```python
from build123d import *

# Parameters (mm, degrees)
F0_W        = 600
F0_H        = 700
F1_DEPTH    = 800
F2_W        = 700
F2_H        = 80
F3_DEPTH    = 25
F5_DEPTH    = 50
F6_T1_DEPTH = 120
F6_T4_ANGLE = 180
F6_T6_ANGLE = 180
F7_W        = 40
F7_H        = 110
F8_DEPTH    = 25
F9_R        = 4.99999
F10_W       = 630
F10_H       = 700
F11_DEPTH   = 25


# Not quite as in the source:
# - a fillet or chamfer that OpenCascade refuses, or shapes differently, is made with other operations: its cross-section is extruded or revolved along the edge and cut away or added
# - a fillet or chamfer is up to 0.001 mm smaller than in the source, because OpenCascade refuses the exact size


with BuildPart() as f1:
    # F0 (on Top) → F1 (new body)
    with BuildSketch(Plane.XY):
        Rectangle(F0_W, F0_H)
    extrude(amount=F1_DEPTH)

    # F2 (on face) → F3 (cut)
    with BuildSketch(Plane.YZ.offset(300)):
        with Locations((0, 40)):
            Rectangle(F2_W, F2_H)
    extrude(amount=-F3_DEPTH, mode=Mode.SUBTRACT)

    # F4 (on face) → F5 (join)
    with BuildSketch(Plane.YZ.offset(300)):
        with BuildLine():
            ThreePointArc((-320, 750), (-323.5355339059, 748.5355339059), (-325, 745))
            Line((-325, 745), (-325, 625))
            ThreePointArc((-325, 625), (-323.5355339059, 621.4644660941), (-320, 620))
            ThreePointArc((-320, 620), (-316.4644660941, 621.4644660941), (-315, 625))
            Line((-315, 625), (-315, 745))
            ThreePointArc((-315, 745), (-316.4644660941, 748.5355339059), (-320, 750))
        make_face()
    extrude(amount=F5_DEPTH)

    # F6: fillet of radius 5 on 4 edges, made by hand

    # F6_s2 → F6_t1 (cut)
    with BuildSketch(Plane.XY.offset(625)):
        with BuildLine():
            ThreePointArc((345, -325), (348.5355339059, -323.5355339059), (350, -320))
            Line((350, -320), (350, -325))
            Line((350, -325), (345, -325))
        make_face()
        with BuildLine():
            ThreePointArc((345, -315), (348.5355339059, -316.4644660941), (350, -320))
            Line((350, -320), (350, -315))
            Line((350, -315), (345, -315))
        make_face()
    extrude(amount=F6_T1_DEPTH, mode=Mode.SUBTRACT)

    # F6_s3 → F6_t4 (revolve, cut)
    with BuildSketch(Plane.XY.offset(745)):
        with BuildLine():
            ThreePointArc((345, -325), (348.5355339059, -323.5355339059), (350, -320))
            Line((350, -320), (350, -325))
            Line((350, -325), (345, -325))
        make_face()
    revolve(axis=Axis((350, -320, 745), (-1, 0, 0)), revolution_arc=F6_T4_ANGLE, mode=Mode.SUBTRACT)

    # F6_s5 → F6_t6 (revolve, cut)
    with BuildSketch(Plane.XY.offset(625)):
        with BuildLine():
            ThreePointArc((345, -315), (348.5355339059, -316.4644660941), (350, -320))
            Line((350, -320), (350, -315))
            Line((350, -315), (345, -315))
        make_face()
    revolve(axis=Axis((350, -320, 625), (-1, 0, 0)), revolution_arc=F6_T6_ANGLE, mode=Mode.SUBTRACT)

    # F7 (on face) → F8 (cut)
    with BuildSketch(Plane(origin=(0, -315, 0), x_dir=(-1, 0, 0), z_dir=(0, 1, 0))):
        with Locations((-320, 685)):
            Rectangle(F7_W, F7_H)
    extrude(amount=-F8_DEPTH, mode=Mode.SUBTRACT)

    # F9 (radius 5 in the source; OpenCascade refuses exactly that, so slightly less here)
    f9_edges = [f1.edges().sort_by_distance(p)[0] for p in [
        (320, -315, 740),
        (340, -315, 685),
        (320, -315, 630),
        (320, -325, 740),
        (340, -325, 685),
        (320, -325, 630),
    ]]
    fillet(f9_edges, radius=F9_R)

    # F10 (on face) → F11 (join)
    with BuildSketch(Plane.XY.offset(800)):
        with Locations((15, 0)):
            Rectangle(F10_W, F10_H)
    extrude(amount=F11_DEPTH)


solid = f1.part
```
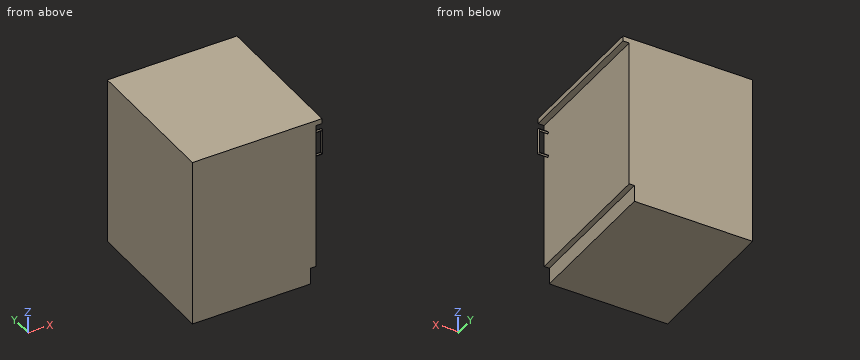
Geometry check sheet. Reference: the model listing, model coordinates, mm. Coordinates: 2 decimals unless noted, no trailing zeros. Order: outer loops, then holes, each group sorted by start corner. A loop starts at its lowest first (then second) coordinate and runs counter-clockwise, first axis right, second up.
Item 1: Section check C-C (z = 336.5). Enter the section's corners in (x, y), plus the area to 3 significant figures.
Item 2: Scan lines: line 1 along X through (y, z) = (-244, 744); line 2 along Z through (x, y) = (297, -273.5); line 3 along X through (y, z) = (-28.5, 79). Record each from-to range of solid material in increasing order.
Item 3: Section check B-B (y = -62). Enter the section's corners in (x, z), plus the area to 3 significant figures.
Item 4: Depth check by flat-ended pin: pin 1 (9 mm diameter, centred on x = 307.5, y = 37.5, fed in from -Z); pin 2 (22.5 mm diameter, centred on x = 314, z = 680.5, fed in from +Y); pin 3 (5 mm diameter, centred on y = -83, z = 280.5, fed in from +X). Enter the tip coordinate at first touch or a pass-through.
Check sheet entries:
1. outline: (-300, -350) - (300, -350) - (300, 350) - (-300, 350) - close
1. area: 420,000 mm2
2. line 1: x = -300 to 300
2. line 2: z = 80 to 825
2. line 3: x = -300 to 275
3. outline: (-300, 0) - (275, 0) - (275, 80) - (300, 80) - (300, 800) - (330, 800) - (330, 825) - (-300, 825) - close
3. area: 494,000 mm2
4. pin 1: stops at z = 800
4. pin 2: passes through
4. pin 3: stops at x = 300
